from build123d import *

# Parameters (mm, degrees)
CROQUIS1_W              = 42.3
CROQUIS1_H              = 42.3
CROQUIS1_R              = 12.5
CROQUIS1_R_2            = 2
SALIENTE_EXTRUIR2_DEPTH = 8
CROQUIS3_W              = 75
CROQUIS3_H              = 80
CROQUIS3_R              = 3
CROQUIS3_W_2            = 20
CROQUIS3_H_2            = 15
SALIENTE_EXTRUIR3_DEPTH = 3
REDONDEO1_R             = 4
REDONDEO3_R             = 6


with BuildPart() as part:
    # Croquis1 → Saliente-Extruir2 (new body)
    with BuildSketch(Plane.XY):
        Rectangle(CROQUIS1_W, CROQUIS1_H)
        Circle(CROQUIS1_R, mode=Mode.SUBTRACT)
        with Locations((-15.5, 15.5)):
            Circle(CROQUIS1_R_2, mode=Mode.SUBTRACT)
        with Locations((15.5, 15.5)):
            Circle(CROQUIS1_R_2, mode=Mode.SUBTRACT)
        with Locations((15.5, -15.5)):
            Circle(CROQUIS1_R_2, mode=Mode.SUBTRACT)
        with Locations((-15.5, -15.5)):
            Circle(CROQUIS1_R_2, mode=Mode.SUBTRACT)
    saliente_extruir2 = extrude(amount=SALIENTE_EXTRUIR2_DEPTH)

    # Croquis3 → Saliente-Extruir3 (add)
    with BuildSketch(Plane(origin=(0, 21.15, 0), x_dir=(1, 0, 0), z_dir=(0, 1, 0))):
        with Locations((0, 32)):
            Rectangle(CROQUIS3_W, CROQUIS3_H)
        with Locations((-29.5, 0)):
            Circle(CROQUIS3_R, mode=Mode.SUBTRACT)
        with Locations((29.5, 0)):
            Circle(CROQUIS3_R, mode=Mode.SUBTRACT)
        with Locations((0, 32)):
            Rectangle(CROQUIS3_W_2, CROQUIS3_H_2, mode=Mode.SUBTRACT)
    saliente_extruir3 = extrude(amount=SALIENTE_EXTRUIR3_DEPTH)

    # Simetría10: Saliente-Extruir3 across plane
    add(saliente_extruir3.mirror(Plane(origin=(0, 0, -72), x_dir=(1, 0, 0), z_dir=(0, 0, -1))))

    # Simetría12: Saliente-Extruir2 across plane
    add(saliente_extruir2.mirror(Plane(origin=(0, 0, -72), x_dir=(1, 0, 0), z_dir=(0, 0, -1))))

    # Redondeo1
    redondeo1_edges = [part.edges().sort_by_distance(p)[0] for p in [
        (21.15, -21.15, 4),
        (-21.15, -21.15, 4),
        (-21.15, -21.15, -148),
        (21.15, -21.15, -148),
    ]]
    fillet(redondeo1_edges, radius=REDONDEO1_R)

    # Redondeo3
    redondeo3_edges = [part.edges().sort_by_distance(p)[0] for p in [
        (-37.5, 22.65, 8),
        (37.5, 22.65, 8),
        (-37.5, 22.65, -152),
        (37.5, 22.65, -152),
    ]]
    fillet(redondeo3_edges, radius=REDONDEO3_R)


solid = part.part
Design review of the part built by this model. Coordinates are the model's own, in mm. A direction names the side the tool comes from. Give positions to 0.01 mm unless a question says otherwise; leave off trailing zeros. Loops run counter-clockwise (first coordinate to the right, second up) from the corner with the lowest first, then second, coordinate; pieces in that order, holes last. Notation, with made-up numbers: M 22.5,4.5 L 28.5,4.5 A31 ccw 28.5,30.5 Z; hole C 36,82.5 d9. An arc over 180 degrees is marked long. Write item = value, one per line.
Q1. We need section A-A (x = 0). Give the boundary of the cut face in (y, z).
Output values:
outline = M -21.15,-152 L -12.5,-152 L -12.5,-144 L -21.15,-144 Z; M -21.15,0 L -12.5,0 L -12.5,8 L -21.15,8 Z; M 12.5,-152 L 24.15,-152 L 24.15,-119.5 L 21.15,-119.5 L 21.15,-144 L 12.5,-144 Z; M 12.5,0 L 21.15,0 L 21.15,-24.5 L 24.15,-24.5 L 24.15,8 L 12.5,8 Z; M 21.15,-104.5 L 24.15,-104.5 L 24.15,-39.5 L 21.15,-39.5 Z
Q2. To check wall thickness, follow line 1 (Y direction, x = -15.5, z = -147.5); line 2 (X direction, y = 22.3, z = 0); line 3 (Z direction, x = -29.5, y = 22.9). State the ranges of each line that lie inside material, in increasing order. Write a range as [from, to].
Output values:
line_1 = [-21.15, -17.5], [-13.5, 13.5], [17.5, 24.15]
line_2 = [-37.5, -32.5], [-26.5, 26.5], [32.5, 37.5]
line_3 = [-152, -147], [-141, -3], [3, 8]
Q3. Insertion check: pin 1 (3.5 mm diameter, centred on x = -15.5, y = -15.5, fed in from -Z); pin 2 (4 mm diameter, centred on y = -5, z = 4, fed in from -X); pin 3 (9 mm diameter, centred on y = -4.5, z = -148.5, fed in from +X); pin 4 (1.5 mm diameter, centred on x = -27.5, z = -63.5, fed in from -Y). Each pin has a flat end and moves straight along its axis. Give the tip position at first contact, or say it passes through.
Output values:
pin_1 = through
pin_2 = -21.15
pin_3 = 21.15
pin_4 = 21.15
Q4. Draft analysis for pull direction Z (two halves, no side actions). For faces 4 (the flat face through (7, 11, -152)), 5 (the cylindrical face through (20.009, -19.947, 4.056)), 6 (the flat face through (0, 23, -24.5)), state which applies: +Z half, -Z half, draft (parallel to the pull), parting line (faces both ways), or undercut.
Output values:
face_4 = -Z half
face_5 = draft
face_6 = undercut
Q5. We need section B-B (x = 29.5). Give the boundary of the cut face in (y, z), plus the area to 3 significant figures.
Output values:
outline = M 21.15,-152 L 24.15,-152 L 24.15,-147 L 21.15,-147 Z; M 21.15,-141 L 24.15,-141 L 24.15,-3 L 21.15,-3 Z; M 21.15,3 L 24.15,3 L 24.15,8 L 21.15,8 Z
area = 444 mm^2
Q6. We need section D-D (y = 15.5). Give the boundary of the cut face in (x, z).
Output values:
outline = M -21.15,-152 L -17.5,-152 L -17.5,-144 L -21.15,-144 Z; M -21.15,0 L -17.5,0 L -17.5,8 L -21.15,8 Z; M -13.5,-152 L 13.5,-152 L 13.5,-144 L -13.5,-144 Z; M -13.5,0 L 13.5,0 L 13.5,8 L -13.5,8 Z; M 17.5,-152 L 21.15,-152 L 21.15,-144 L 17.5,-144 Z; M 17.5,0 L 21.15,0 L 21.15,8 L 17.5,8 Z
Q7. For faces 1 (the flat face through (-21.15, 2, 4)), 2 (the cylindrical face through (15.24, 17.483, -147.944)), 3 (the flat face through (10, 23, -32)), list the 3-axis set-ups (+Z, -Z, +X, -X, +Y, -Y) from which the entire face can be reached by the end or side of a thin tool; tool diameter is ignored.
Output values:
face_1 = +Z, -Z, -X, -Y
face_2 = +Z, -Z
face_3 = +Y, -Y
Q8. We need section C-C (y = 0). Give the boundary of the cut face in (x, z).
Output values:
outline = M -21.15,-152 L -12.5,-152 L -12.5,-144 L -21.15,-144 Z; M -21.15,0 L -12.5,0 L -12.5,8 L -21.15,8 Z; M 12.5,-152 L 21.15,-152 L 21.15,-144 L 12.5,-144 Z; M 12.5,0 L 21.15,0 L 21.15,8 L 12.5,8 Z
